Geometry: final body of the model. Coordinates: model frame, mm. A direction names the side the tool comes from. Coordinates: 2 decimals unless noted, no trailing zeros. Order: outer loops, then holes, each group sorted by start corner. A loop starts at its lowest first (then second) coordinate and runs counter-clockwise, first axis right, second up. Notation, with made-up numbers: M 20.5,76.25 L 57.5,76.25 A23 cw 57.5,113.25 Z; hole C 82,40 d2. An arc over 180 degrees is marked long. Write item = value, one per line.
from build123d import *

# Parameters (mm, degrees)
F1_DEPTH       = 38.1
F2_DEPTH       = 711.2
F0_W           = 654.05
F0_H           = 222.25
F3_DEPTH       = 711.2
F4_W           = 673.1
F4_H           = 139.7
F4_W_2         = 635
F4_H_2         = 228.6
F5_DEPTH       = 406.401
F0_W_2         = 19.05
F0_H_2         = 19.05
F6_DEPTH       = 38.1
F7_DEPTH       = 711.2
F8_W           = 476.25
F8_H           = 139.7
F8_W_2         = 241.3
F8_H_2         = 228.6
F9_DEPTH       = 406.4
F10_W          = 203.2
F10_H          = 228.6
F11_DEPTH      = 609.6
F11_DEPTH_BACK = 266.7
F13_START      = -152.4
F12_W          = 38.1
F12_H          = 552.45
F13_DEPTH      = 558.8


with BuildPart() as f1:
    # F0 (on Top) → F1 (new body)
    with BuildSketch(Plane.XY):
        Polygon((285.75, 184.15), (304.8, 184.15), (304.8, 406.4), (-285.75, 406.4), (-285.75, -387.35), (285.75, -387.35), (285.75, 165.1), align=None)
        with BuildLine():
            Line((-266.7, -406.4), (266.7, -406.4))
            ThreePointArc((266.7, -406.4), (293.6407683632, -395.2407683632), (304.8, -368.3))
            Line((304.8, -368.3), (304.8, 165.1))
            Line((304.8, 165.1), (285.75, 165.1))
            Line((285.75, 165.1), (285.75, -387.35))
            Line((285.75, -387.35), (-285.75, -387.35))
            Line((-285.75, -387.35), (-285.75, 406.4))
            Line((-285.75, 406.4), (-304.8, 406.4))
            Line((-304.8, 406.4), (-304.8, -368.3))
            ThreePointArc((-304.8, -368.3), (-293.6407683632, -395.2407683632), (-266.7, -406.4))
        make_face()
    extrude(amount=F1_DEPTH)



with BuildPart() as f2:
    # F0 (on Top) → F2 (new body)
    with BuildSketch(Plane.XY):
        Polygon((285.75, 184.15), (304.8, 184.15), (304.8, 406.4), (-285.75, 406.4), (-285.75, -387.35), (285.75, -387.35), (285.75, 165.1), align=None)
    extrude(amount=-F2_DEPTH)


with BuildPart() as f3:
    # F0 (on Top) → F3 (new body)
    with BuildSketch(Plane.XY):
        with Locations((631.825, 295.275)):
            Rectangle(F0_W, F0_H)
        Polygon((304.8, 184.15), (304.8, 165.1), (305.019557476, 165.1), (977.9, 165.1), (977.9, 406.4), (958.85, 406.4), (958.85, 184.15), align=None)
    extrude(amount=-F3_DEPTH)

    # F4 (on Front) → F5 (cut, through all)
    with BuildSketch(Plane.XZ):
        with Locations((641.35, -69.85)):
            Rectangle(F4_W, F4_H)
        with Locations((622.3, -292.1)):
            Rectangle(F4_W_2, F4_H_2)
        with Locations((622.3, -558.8)):
            Rectangle(F4_W_2, F4_H_2)
    extrude(amount=-F5_DEPTH, mode=Mode.SUBTRACT)


with BuildPart() as f1_1:
    add(f1.part)

    add(f2.part)  # F6 merges F2
    # F0 (on Top) → F6 (join)
    with BuildSketch(Plane.XY):
        with Locations((295.275, 174.625)):
            Rectangle(F0_W_2, F0_H_2)
    extrude(amount=F6_DEPTH)


    add(f3.part)  # F7 merges F3
    # F0 (on Top) → F7 (join)
    with BuildSketch(Plane.XY):
        with Locations((295.275, 174.625)):
            Rectangle(F0_W_2, F0_H_2)
    extrude(amount=-F7_DEPTH)

    # F8 (on Right) → F9 (cut, symmetric)
    with BuildSketch(Plane.YZ):
        with Locations((-111.125, -69.85)):
            Rectangle(F8_W, F8_H)
        with Locations((247.65, -69.85)):
            Rectangle(F8_W_2, F8_H)
        with Locations((-111.125, -292.1)):
            Rectangle(F8_W, F8_H_2)
        with Locations((-111.125, -558.8)):
            Rectangle(F8_W, F8_H_2)
    extrude(amount=F9_DEPTH, both=True, mode=Mode.SUBTRACT)

    # F10 (on Right) → F11 (cut, two sides)
    with BuildSketch(Plane.YZ) as f11_sk:
        with Locations((266.7, -292.1)):
            Rectangle(F10_W, F10_H)
        with Locations((266.7, -558.8)):
            Rectangle(F10_W, F10_H)
    extrude(amount=-F11_DEPTH, mode=Mode.SUBTRACT)
    extrude(f11_sk.sketch, amount=F11_DEPTH_BACK, mode=Mode.SUBTRACT)

    # F12 (on Top) → F13 (join)
    with BuildSketch(Plane.XY.offset(F13_START)):
        with Locations((0, -111.125)):
            Rectangle(F12_W, F12_H)
    extrude(amount=-F13_DEPTH)


solid = f1_1.part
1) Section D-D, the plane y = -280. Return loops of the section in (x, z), and give its area (3 significant figures).
Numbers:
outline = M -304.8,0 L 304.8,0 L 304.8,38.1 L -304.8,38.1 Z; M -285.75,-711.2 L 285.75,-711.2 L 285.75,-673.1 L 19.05,-673.1 L 19.05,-444.5 L 285.75,-444.5 L 285.75,-406.4 L 19.05,-406.4 L 19.05,-177.8 L 285.75,-177.8 L 285.75,-139.7 L -285.75,-139.7 L -285.75,-177.8 L -19.05,-177.8 L -19.05,-406.4 L -285.75,-406.4 L -285.75,-444.5 L -19.05,-444.5 L -19.05,-673.1 L -285.75,-673.1 Z
area = 106,000 mm²
2) Pin query (flat end, axial travel): pin 1 (1 mm diameter, centred on x = 738.5, y = 274.5, fed in from +Z); pin 2 (4 mm diameter, centred on x = 605.5, z = -444, fed in from -Y). Return the tip coordinate at first contact, or that it passes through.
Numbers:
pin_1 = -139.7
pin_2 = 165.1
3) Section C-C, the plane x = 551.5. Return loops of the section in (y, z), and give its area (3 significant figures).
Numbers:
outline = M 165.1,-711.2 L 406.4,-711.2 L 406.4,-673.1 L 165.1,-673.1 Z; M 165.1,-444.5 L 406.4,-444.5 L 406.4,-406.4 L 165.1,-406.4 Z; M 165.1,-177.8 L 406.4,-177.8 L 406.4,-139.7 L 165.1,-139.7 Z
area = 27,600 mm²
4) Section B-B, the plane z = -99.5. Return loops of the section in (x, y).
Numbers:
outline = M -285.75,-387.35 L 285.75,-387.35 L 285.75,-349.25 L -285.75,-349.25 Z; M -285.75,368.3 L 304.8,368.3 L 304.8,406.4 L -285.75,406.4 Z
5) Set-up query: faces 1 (the face through (-285.75, 11, -407)), 2 (the face through (-4, -387.35, -351)), 3 (the face through (-6, 368.3, -560)), 4 (the face through (-4, -349.25, -71)). Return all of +Z, -Z, +X, -X, +Y, -Y with unobstructed straight access to the full face (end or side cutting, diameter ignored); none if empty.
Numbers:
face_1 = -Z, -X, +Y, -Y
face_2 = -Z, +X, -X, -Y
face_3 = -X
face_4 = +X, -X
6) Line query: L1, parallel to Y at x = -186.5, z = -223; L2, parallel to Z at x = 168, y = -281; L3, parallel to X at y = 238, z = -533. Output: solid intervals per line, ascending.
Numbers:
L1 = -387.35 to -349.25, 127 to 165.1, 368.3 to 406.4
L2 = -711.2 to -673.1, -444.5 to -406.4, -177.8 to -139.7, 0 to 38.1
L3 = 266.7 to 304.8, 939.8 to 977.9
7) Mould query, pull axis X, two halves, no side actions, for faces 5 (the face through (-293.94, -394.94, 18.78)), 6 (the face through (-6, 265, -406.4)), 7 (the face through (939.8, 284, -560)), 8 (the face through (293.34, -395.54, 18.78)). Classes: pulls with the +X half, pulls with the -X half, needs draft (parallel to the pull), parting line crosses it, or undercut.
Numbers:
face_5 = pulls with the -X half
face_6 = needs draft
face_7 = undercut
face_8 = pulls with the +X half
8) Section A-A, the plane y = 302. Return loops of the section in (x, z), and give its area (4 significant figures).
Numbers:
outline = M -304.8,0 L 304.8,0 L 304.8,38.1 L -304.8,38.1 Z; M -285.75,-711.2 L 977.9,-711.2 L 977.9,-139.7 L -285.75,-139.7 L -285.75,-177.8 L 266.7,-177.8 L 266.7,-406.4 L -285.75,-406.4 L -285.75,-444.5 L 266.7,-444.5 L 266.7,-673.1 L -285.75,-673.1 Z; hole M 304.8,-673.1 L 939.8,-673.1 L 939.8,-444.5 L 304.8,-444.5 Z; hole M 304.8,-406.4 L 939.8,-406.4 L 939.8,-177.8 L 304.8,-177.8 Z
area = 202,500 mm²
